Verification items for the finished model (mm, model axes). Face numbers are marked on the shaded views. A direction names the side the tool comes from. Round coordinates to 2 decimals unless told otherwise and drop trailing zeros. Loops run counter-clockwise (first coordinate to the right, second up) from the corner with the lowest first, then second, coordinate; pieces in that order, holes last. Notation, with made-up numbers: M 88,49 L 146,49 A17 ccw 146,66 Z; hole C 37.5,46.25 d10. An arc over 180 degrees is marked long. One line per item, written item: value.
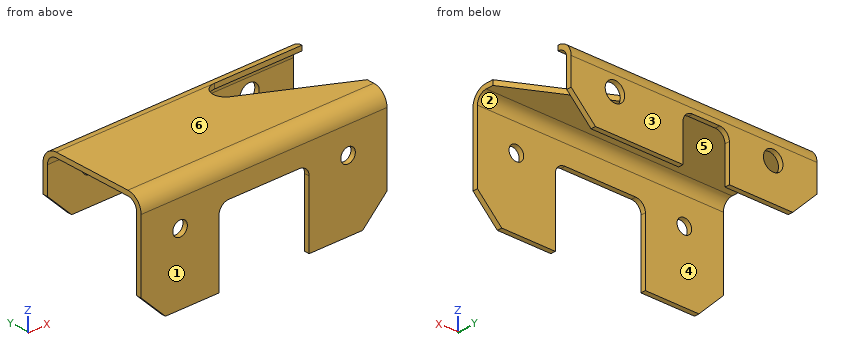
from build123d import *

# Parameters (mm, degrees)
BASE_FLANGE1_DEPTH = 160.3375
CUT_EXTRUDE1_DEPTH = 3.175
CUT_EXTRUDE2_DEPTH = 3.175
CUT_EXTRUDE3_DEPTH = 3.175
CUT_EXTRUDE4_DEPTH = 3.175
CUT_EXTRUDE5_DEPTH = 3.175
CUT_EXTRUDE6_DEPTH = 3.175
SKETCH12_R         = 6.35
CUT_EXTRUDE7_DEPTH = 3.175
SKETCH13_R         = 4.7625
CUT_EXTRUDE8_DEPTH = 3.175
CUT_EXTRUDE9_DEPTH = 3.175


# Sheet-metal steps are written as plain solids
with BuildPart() as part:
    # Sketch1 → Base-Flange1 (new body)
    with BuildSketch(Plane(origin=(0, 0, 0), x_dir=(0, 0, -1), z_dir=(1, 0, 0))):
        with BuildLine():
            Line((71.4375, 0), (9.525, 0))
            ThreePointArc((9.525, 0), (2.789807909, 2.789807909), (0, 9.525))
            Line((0, 9.525), (0, 61.11875))
            ThreePointArc((0, 61.11875), (2.789807909, 67.853942091), (9.525, 70.64375))
            Line((9.525, 70.64375), (42.8625, 70.64375))
            Line((42.8625, 70.64375), (42.8625, 67.46875))
            Line((42.8625, 67.46875), (9.525, 67.46875))
            ThreePointArc((9.525, 67.46875), (5.034871939, 65.608878061), (3.175, 61.11875))
            Line((3.175, 61.11875), (3.175, 9.525))
            ThreePointArc((3.175, 9.525), (5.034871939, 5.034871939), (9.525, 3.175))
            Line((9.525, 3.175), (71.4375, 3.175))
            Line((71.4375, 3.175), (71.4375, 0))
        make_face()
    extrude(amount=-BASE_FLANGE1_DEPTH)

    # Sketch6 → Cut-Extrude1 (cut)
    with BuildSketch(Plane(origin=(0, 3.175, 0), x_dir=(1, 0, 0), z_dir=(0, 1, 0))):
        with BuildLine():
            Line((-50.8, 71.4375), (-50.8, 28.575))
            ThreePointArc((-50.8, 28.575), (-52.659871939, 24.084871939), (-57.15, 22.225))
            Line((-57.15, 22.225), (-103.1875, 22.225))
            ThreePointArc((-103.1875, 22.225), (-107.677628061, 24.084871939), (-109.5375, 28.575))
            Line((-109.5375, 28.575), (-109.5375, 71.4375))
            Line((-109.5375, 71.4375), (-50.8, 71.4375))
        make_face()
    extrude(amount=-CUT_EXTRUDE1_DEPTH, mode=Mode.SUBTRACT)

    # Sketch7 → Cut-Extrude2 (cut)
    with BuildSketch(Plane(origin=(0, 3.175, 0), x_dir=(1, 0, 0), z_dir=(0, 1, 0))):
        Polygon((0, 71.4375), (-15.875, 71.4375), (0, 55.5625), align=None)
    extrude(amount=-CUT_EXTRUDE2_DEPTH, mode=Mode.SUBTRACT)

    # Sketch8 → Cut-Extrude3 (cut)
    with BuildSketch(Plane(origin=(0, 3.175, 0), x_dir=(1, 0, 0), z_dir=(0, 1, 0))):
        Polygon((-160.3375, 71.4375), (-144.4625, 71.4375), (-160.3375, 55.5625), align=None)
    extrude(amount=-CUT_EXTRUDE3_DEPTH, mode=Mode.SUBTRACT)

    # Sketch9 → Cut-Extrude4 (cut)
    with BuildSketch(Plane(origin=(0, 70.64375, 0), x_dir=(1, 0, 0), z_dir=(0, 1, 0))):
        Polygon((-160.3375, 42.8625), (-144.4625, 42.8625), (-160.3375, 26.9875), align=None)
    extrude(amount=-CUT_EXTRUDE4_DEPTH, mode=Mode.SUBTRACT)

    # Sketch10 → Cut-Extrude5 (cut)
    with BuildSketch(Plane(origin=(0, 70.64375, 0), x_dir=(1, 0, 0), z_dir=(0, 1, 0))):
        Polygon((0, 42.8625), (-15.875, 42.8625), (0, 26.9875), align=None)
    extrude(amount=-CUT_EXTRUDE5_DEPTH, mode=Mode.SUBTRACT)

    # Sketch11 → Cut-Extrude6 (cut)
    with BuildSketch(Plane.XY):
        with BuildLine():
            Line((0, 61.11875), (-57.15, 61.11875))
            ThreePointArc((-57.15, 61.11875), (-64.857648322, 55.07757898), (-60.83283134, 46.149844766))
            Line((-60.83283134, 46.149844766), (0, 14.2875))
            Line((0, 14.2875), (0, 61.11875))
        make_face()
    extrude(amount=-CUT_EXTRUDE6_DEPTH, mode=Mode.SUBTRACT)

    # Sketch12 → Cut-Extrude7 (cut)
    with BuildSketch(Plane(origin=(0, 70.64375, 0), x_dir=(1, 0, 0), z_dir=(0, 1, 0))):
        with Locations(Location((-28.575, 19.05, 0), (0, 0, 270))):
            Circle(SKETCH12_R)
        with Locations(Location((-131.7625, 19.05, 0), (0, 0, 270))):
            Circle(SKETCH12_R)
    extrude(amount=-CUT_EXTRUDE7_DEPTH, mode=Mode.SUBTRACT)

    # Sketch13 → Cut-Extrude8 (cut)
    with BuildSketch(Plane(origin=(0, 3.175, 0), x_dir=(1, 0, 0), z_dir=(0, 1, 0))):
        with Locations(Location((-25.4, 26.614015176, 0), (0, 0, 270))):
            Circle(SKETCH13_R)
        with Locations(Location((-134.9375, 26.614015176, 0), (0, 0, 270))):
            Circle(SKETCH13_R)
    extrude(amount=-CUT_EXTRUDE8_DEPTH, mode=Mode.SUBTRACT)

    # Sketch14 → Cut-Extrude9 (cut)
    with BuildSketch(Plane(origin=(0, 70.64375, 0), x_dir=(1, 0, 0), z_dir=(0, 1, 0))):
        with BuildLine():
            Line((-72.9615, 42.8625), (-72.9615, 19.05))
            ThreePointArc((-72.9615, 19.05), (-74.821371939, 14.559871939), (-79.3115, 12.7))
            Line((-79.3115, 12.7), (-96.8375, 12.7))
            ThreePointArc((-96.8375, 12.7), (-101.327628061, 14.559871939), (-103.1875, 19.05))
            Line((-103.1875, 19.05), (-103.1875, 42.8625))
            Line((-103.1875, 42.8625), (-72.9615, 42.8625))
        make_face()
    extrude(amount=-CUT_EXTRUDE9_DEPTH, mode=Mode.SUBTRACT)


solid = part.part
(1) Sectioned sample at B-B on x = -25.4. Count the separate pieces of the cut face and the enclosed holes in it, and give its area (3 significant figures).
Completed:
separate pieces: 4
enclosed holes: 0
area: 374 mm^2
(2) Sectioned sample at D-D on z = -16. Enter the section's corners in (x, y) (1 decimal), and give its area (3 significant figures).
Completed:
outline: M -160.3,0 L 0,0 L 0,3.2 L -160.3,3.2 Z; M -160.3,67.5 L -137.3,67.5 L -137.3,70.6 L -160.3,70.6 Z; M -126.2,67.5 L -102.4,67.5 L -102.4,70.6 L -126.2,70.6 Z; M -73.7,67.5 L -34.1,67.5 L -34.1,70.6 L -73.7,70.6 Z; M -23,67.5 L 0,67.5 L 0,70.6 L -23,70.6 Z
area: 856 mm^2
(3) Depth check by flat-ended pin: pin 1 Ø1.6 at (x, y) = (-126, 68.5) entering from -Z; pin 2 Ø2.5 at (x, z) = (-27, -2) entering from -Y; pin 3 Ø15.5 at (x, y) = (-68.5, 29.5) entering from -Z (3 decimals); pin 4 Ø10 at (y, z) = (25, -10.5) entering from -X. Enter the tip coordinate at first touch or a pass-through.
Completed:
pin 1: stops at z = -42.86
pin 2: stops at y = 2.36
pin 3: stops at z = -3.175
pin 4: passes through
(4) Sectioned sample at A-A on z = -46. Enter the section's corners in (x, y) (1 decimal), and give its area (3 significant figures).
Completed:
outline: M -160.3,0 L -109.5,0 L -109.5,3.2 L -160.3,3.2 Z; M -50.8,0 L 0,0 L 0,3.2 L -50.8,3.2 Z
area: 323 mm^2
(5) Tool access check on the marked faces 5 and 6. Record the directions out of +Z, -Z, +X, -X, +Y, -Y that give a thin tool (end or side, any length) a straight path to the whole face; none if there is none.
Completed:
face 5: -Z, +X, -X
face 6: +Z, +X, -X, +Y, -Y
(6) Mould release check, pull along Y, two halves, no side actions. Record for the marked faces 1, 2, 3 and 4: +Y half, -Y half, draft (parallel to the pull), parting line (faces both ways), or undercut.
Completed:
face 1: -Y half
face 2: undercut
face 3: +Y half
face 4: undercut
(7) Thickness scan on L1, parallel to Y at x = -24.5, z = -37 (3 decimals); L2, parallel to Y at x = -82, z = -17 (3 decimals); L3, parallel to Z at x = -152, y = 40 (3 decimals). Record the ranges inside material, lowest first. Write a range as from..to.
Completed:
L1: y = 0..3.175, 67.469..70.644
L2: y = 0..3.175
L3: z = -3.175..0
